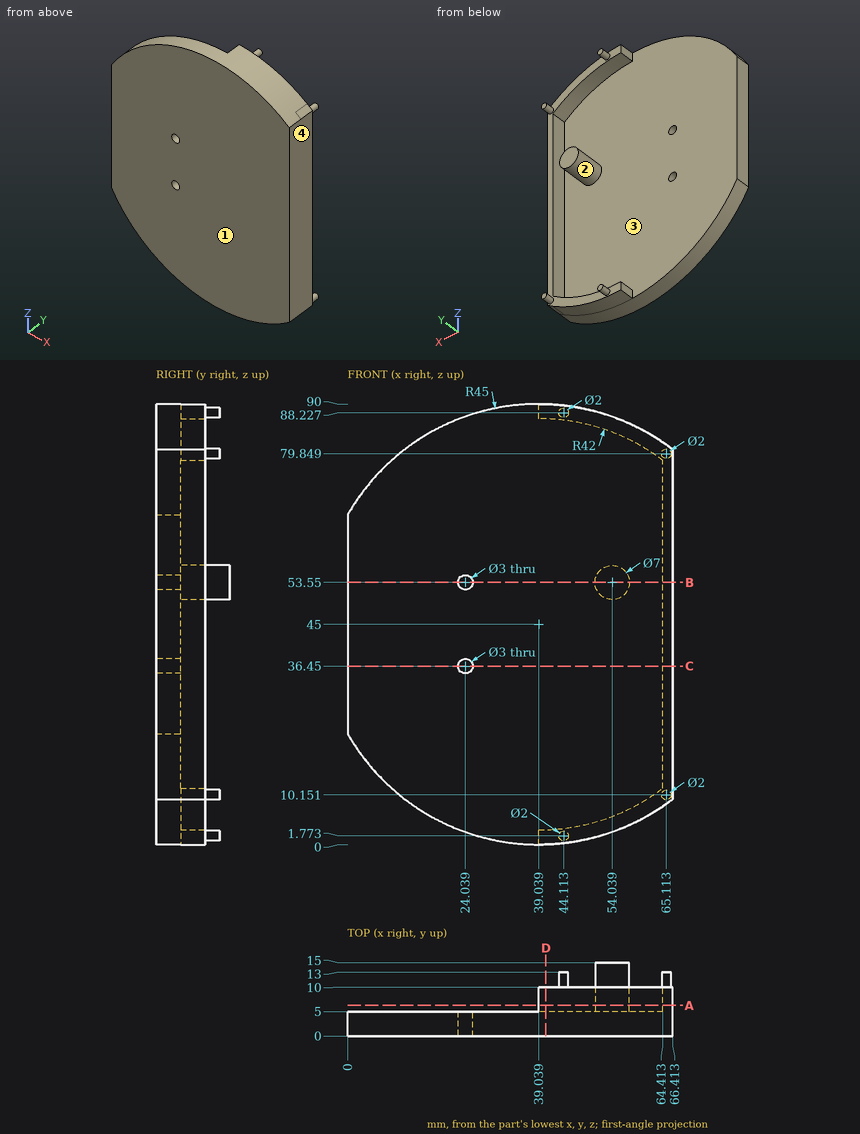
The figure shows three views and two pictorial views of one solid part (mm, origin at its lowest corner). Answer the questions. A direction names the side the tool comes from. Coordinates: 2 decimals unless noted, no trailing zeros. Loops run counter-clockwise (first coordinate to the right, second up) from the corner with the lowest first, then second, coordinate; pieces in that order, holes last. Notation, with made-up numbers: (38, -22.5) - (91, -22.5) arc R11 ccw to (91, -8.5) - close; hole circle Ø9 at (-17, 25). An arc over 180 degrees is marked (long way). Answer in a Markdown table with one row per item.
Q1. Find section D-D on x = 40.5. Write down the section's boundary in (y, z) (1 decimal), plus the area to 3 significant figures.
Here are the results:
| item | result |
|---|---|
| outline | (0, 0) - (10, 0) - (10, 3) - (5, 3) - (5, 87) - (10, 87) - (10, 90) - (0, 90) - close |
| area | 480 mm^2 |
Q2. Find section A-A on y = 6.25. Write down the section's boundary in (x, z), plus the area to 3 significant figures.
Here are the results:
| item | result |
|---|---|
| outline | (39.04, 0) arc R45 ccw to (66.41, 9.28) - (66.41, 80.72) arc R45 ccw to (39.04, 90) - (39.04, 87) arc R42 cw to (64.41, 78.47) - (64.41, 11.53) arc R42 cw to (39.04, 3) - close; circle Ø7 at (54.04, 53.55) |
| area | 347 mm^2 |
Q3. The mould has two halves that part along Z. Classify the marked faces 3 and 4: pulls with the +Z half, pulls with the -Z half, needs draft (parallel to the pull), parting line crosses it, or undercut.
Here are the results:
| item | result |
|---|---|
| face 3 | undercut |
| face 4 | needs draft |
Q4. Find section C-C on z = 36.45. Write down the section's boundary in (x, y).
Here are the results:
| item | result |
|---|---|
| outline | (0, 0) - (22.54, 0) - (22.54, 5) - (0, 5) - close; (25.54, 0) - (66.41, 0) - (66.41, 10) - (64.41, 10) - (64.41, 5) - (25.54, 5) - close |
Q5. Given P1, Ø0.6, axis at x = 44, z = 2, coming from the +Y side; P2, Ø3.5, axis at y = 8.5, z = 1.5, coming from the -X side; P3, Ø4, axis at x = 24.04, z = 36.45, coming from the +Y side, each flat-ended and moving along its own axis, determine where each tip first touches the part or whether it passes through.
Here are the results:
| item | result |
|---|---|
| P1 | stops at y = 13 |
| P2 | stops at x = 39.04 |
| P3 | stops at y = 5 |
Q6. Find section B-B on z = 53.55. Write down the section's boundary in (x, y).
Here are the results:
| item | result |
|---|---|
| outline | (0, 0) - (22.54, 0) - (22.54, 5) - (0, 5) - close; (25.54, 0) - (66.41, 0) - (66.41, 10) - (64.41, 10) - (64.41, 5) - (57.54, 5) - (57.54, 15) - (50.54, 15) - (50.54, 5) - (25.54, 5) - close |
Q7. For the marked faces 1 and 2, determine the directions among +Z, -Z, +X, -X, +Y, -Y from which every point of the face is accessible in a straight line to the end or side of a thin tool.
Here are the results:
| item | result |
|---|---|
| face 1 | +Z, -Z, +X, -X, -Y |
| face 2 | +Y |
Q8. Straight lines are drawn through the part: line 1 along X through (y, z) = (1.75, 53.55); line 2 along Z through (x, y) = (39.5, 5.75); line 3 along Y through (x, z) = (13, 70.5). For each, find the intervals that lie inside material, in ascending order. Write a range as [from, to].
Here are the results:
| item | result |
|---|---|
| line 1 | x = [0, 22.54], [25.54, 66.41] |
| line 2 | z = [0, 3], [87, 90] |
| line 3 | y = [0, 5] |
